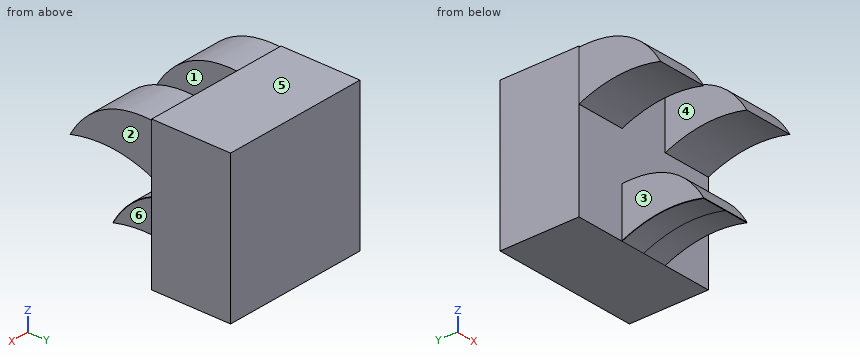
```python
from build123d import *

# Parameters (mm, degrees)
SKETCH_1_W               = 15
SKETCH_1_H               = 15
EXTRUDE_1_DEPTH          = 4
EXTRUDE_2_DEPTH          = 2.5
PATTERN_START            = -7.500040123
PATTERN_SKETCH_2_DEPTH   = 5
PATTERN_START_2          = 2.499959877
PATTERN_SKETCH_2_2_DEPTH = 5
PATTERN_START_3          = -2.500040123
PATTERN_SKETCH_2_3_DEPTH = 5


with BuildPart() as part:
    # 스케치1 → 보스-돌출1 (new, symmetric)
    with BuildSketch(Plane(origin=(0, 0, 0), x_dir=(1, 0, 0), z_dir=(0, 1, 0))):
        Rectangle(SKETCH_1_W, SKETCH_1_H)
    extrude(amount=EXTRUDE_1_DEPTH, both=True)

    # 스케치3 → 보스-돌출2 (add, symmetric)
    with BuildSketch(Plane(origin=(0, 0, 0), x_dir=(0, 0, -1), z_dir=(1, 0, 0))):
        with BuildLine():
            Line((2.5, -4), (7.5, -4))
            add(Edge.make_bspline(
                [(6.837946582, -12.278081575), (5.73941202, -8.009656666), (7.5, -4)],
                knots=[0, 0, 0, 1, 1, 1], degree=2))
            add(Edge.make_bspline(
                [(2.5, -4), (2.152812134, -9.664313578), (6.837946582, -12.278081575)],
                knots=[0, 0, 0, 1, 1, 1], degree=2))
        make_face()
    extrude(amount=EXTRUDE_2_DEPTH, both=True)

    # 스케치 패턴2: read off the stored shape, not the designer's step
    # 스케치 패턴2 outline → 스케치 패턴2 (add)
    with BuildSketch(Plane.YZ.offset(PATTERN_START)):
        with BuildLine():
            Line((-4, 2.400000403), (-4, 7.400000403))
            add(Edge.make_bspline(
                [(-4, 7.400000403), (-9.664313578, 7.747188269), (-12.278081575, 3.062053822)],
                knots=[0, 0, 0, 1, 1, 1], degree=2))
            add(Edge.make_bspline(
                [(-12.278081575, 3.062053822), (-8.009656666, 4.160588383), (-4, 2.400000403)],
                knots=[0, 0, 0, 1, 1, 1], degree=2))
        make_face()
    extrude(amount=PATTERN_SKETCH_2_DEPTH)

    # Pattern Sketch 2 2 outline → Pattern Sketch 2 2 (add)
    with BuildSketch(Plane.YZ.offset(PATTERN_START_2)):
        with BuildLine():
            Line((-4, 2.400000403), (-4, 7.400000403))
            add(Edge.make_bspline(
                [(-4, 7.400000403), (-9.664313578, 7.747188269), (-12.278081575, 3.062053822)],
                knots=[0, 0, 0, 1, 1, 1], degree=2))
            add(Edge.make_bspline(
                [(-12.278081575, 3.062053822), (-8.009656666, 4.160588383), (-4, 2.400000403)],
                knots=[0, 0, 0, 1, 1, 1], degree=2))
        make_face()
    extrude(amount=PATTERN_SKETCH_2_2_DEPTH)

    # Pattern Sketch 2 3 outline → Pattern Sketch 2 3 (add)
    with BuildSketch(Plane.YZ.offset(PATTERN_START_3)):
        with BuildLine():
            add(Edge.make_bspline(
                [(-4, -2.439999597), (-9.664313578, -2.092811731), (-12.278081575, -6.777946178)],
                knots=[0, 0, 0, 1, 1, 1], degree=2))
            add(Edge.make_bspline(
                [(-12.278081575, -6.777946178), (-8.009656666, -5.679411617), (-4, -7.439999597)],
                knots=[0, 0, 0, 1, 1, 1], degree=2))
            Line((-4, -7.439999597), (-4, -2.439999597))
        make_face()
    extrude(amount=PATTERN_SKETCH_2_3_DEPTH)


solid = part.part
```
Work out the finished part from the listing and answer in its coordinate system (mm). Face numbers are marked on the shaded views. A direction names the side the tool comes from. Give positions to 0.01 mm unless a question says otherwise; leave off trailing zeros. Loops run counter-clockwise (first coordinate to the right, second up) from the corner with the lowest first, then second, coordinate; pieces in that order, holes last. Notation, with made-up numbers: (15.25, -33.5) - (51.25, -33.5) arc R18 cw to (51.25, -9.5) - close; hole circle Ø4 at (-13, 70). An arc over 180 degrees is marked (long way). Use CSV: the item, a comma, the result in double quotes. Start each with the question number.
(1) Find section A-A, the plane y = -4.75. Count the separate pieces of the cut face and the enclosed holes in it, plus the area to 3 significant figures.
(2) Each of these flat-tipped pins is pushed along its axis until it touches: pin 1 (2 mm diameter, centred on y = -8.5, z = -4, fed in from +X); pin 2 (1.3 mm diameter, centred on y = -8.5, z = -7, fed in from -X). Where does it stop, or does it pass through?
(3) Find section B-B, the plane z = 0. Determine the outline of the cut face in (x, y).
(4) Determine the mould class of the marked faces 1, 2, 3 and 4 for opening direction X: released by +X, released by -X, zero draft, split by the parting line, or undercut.
(5) Find the intervals of material crossed by L1, parallel to X at y = -5, z = 4; L2, parallel to X at y = -4.75, z = -2.5; L3, parallel to Y at x = 5.5, z = -0.5, in increasing order.
(6) A tool of negligible diameter and unlimited length cuts with its end or side. For the marked faces 5 and 6, from which of +Z, -Z, +X, -X, +Y, -Y can it reach the whole face along a straight path? Write none if from no direction.
Results found:
1,separate pieces,"3"
1,enclosed holes,"0"
1,area,"71.1 mm^2"
2,pin 1,"x = 2.5"
2,pin 2,"x = -2.5"
3,outline,"(-7.5, -4) - (7.5, -4) - (7.5, 4) - (-7.5, 4) - close"
4,face 1,"undercut"
4,face 2,"released by +X"
4,face 3,"released by -X"
4,face 4,"undercut"
5,L1,"-7.5 to -2.5, 2.5 to 7.5"
5,L2,"-2.5 to 2.5"
5,L3,"-4 to 4"
6,face 5,"+Z, +X, -X, +Y, -Y"
6,face 6,"-Z, +X, -Y"
